Could you check a few things on this model? Use its own coordinates, in mm. Face numbers are marked on the shaded views. A direction names the side the tool comes from. Give positions to 0.01 mm unless a question says otherwise; leave off trailing zeros. Write each loop counter-clockwise with the first axis right and the second up, starting at its lowest first coordinate (ties: lowest second). Pieces come first, ordered by that corner, then holes. Notation, with made-up numbers: (-4, 16.5) - (32, 16.5) arc R10 ccw to (32, 24.5) - close; hole circle Ø2 at (2.25, -33). An arc over 180 degrees is marked (long way). Answer in a Markdown table with one row per item.
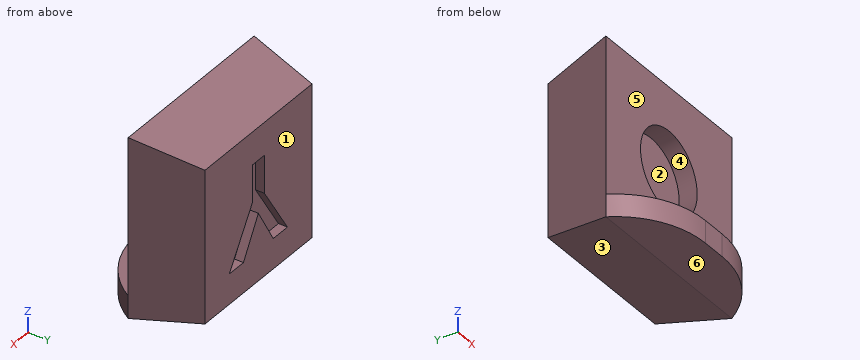
from build123d import *

# Parameters (mm, degrees)
SKETCH1_W               = 8
SKETCH1_H               = 8
BOSS_EXTRUDE1_DEPTH     = 3
CUT_EXTRUDE1_DEPTH      = 12.704699911
CUT_EXTRUDE1_DEPTH_BACK = 12.704699911
CUT_EXTRUDE2_DEPTH      = 11
SKETCH4_R               = 1.8
CUT_EXTRUDE3_DEPTH      = 0.8
SKETCH5_W               = 8
SKETCH5_H               = 1
BOSS_EXTRUDE2_DEPTH     = 2
FILLET1_R               = 4
CUT_EXTRUDE4_DEPTH      = 0.4


with BuildPart() as part:
    # Sketch1 → Boss-Extrude1 (new body)
    with BuildSketch(Plane(origin=(0, 0, 0), x_dir=(1, 0, 0), z_dir=(0, 1, 0))):
        with Locations((4, 4)):
            Rectangle(SKETCH1_W, SKETCH1_H)
    extrude(amount=BOSS_EXTRUDE1_DEPTH)

    # Sketch2 → Cut-Extrude1 (cut, two sides: drawn at the far end of the back side and taken through both)
    with BuildSketch(Plane.XY.offset(-CUT_EXTRUDE1_DEPTH_BACK)):
        Polygon((0, 0), (0.6, 3), (0, 3), align=None)
        Polygon((8, 0), (7.4, 3), (8, 3), align=None)
    extrude(amount=CUT_EXTRUDE1_DEPTH + CUT_EXTRUDE1_DEPTH_BACK, mode=Mode.SUBTRACT)

    # Sketch3 → Cut-Extrude2 (cut)
    with BuildSketch(Plane(origin=(0, 0, 0), x_dir=(0, 0, -1), z_dir=(1, 0, 0))):
        Polygon((0, 0), (0.6, 3), (0, 3), align=None)
        Polygon((8, 3), (7.4, 3), (8, 0), align=None)
    extrude(amount=CUT_EXTRUDE2_DEPTH, mode=Mode.SUBTRACT)

    # Sketch4 → Cut-Extrude3 (cut)
    with BuildSketch(Plane.XZ):
        with Locations(Location((4, -3.75, 0), (0, 0, 270))):
            Circle(SKETCH4_R)
    extrude(amount=-CUT_EXTRUDE3_DEPTH, mode=Mode.SUBTRACT)

    # Sketch5 → Boss-Extrude2 (add)
    with BuildSketch(Plane.XZ):
        with Locations((4, -7.5)):
            Rectangle(SKETCH5_W, SKETCH5_H)
    extrude(amount=BOSS_EXTRUDE2_DEPTH)

    # Fillet1
    # the kernel refuses this fillet: 4 mm, written as the material it takes off along each edge
    with BuildSketch(Plane(origin=(8, -2, -16.660254038), x_dir=(0, 1, 0), z_dir=(0, 0, 1)), Plane(origin=(0, -2, 1.660254038), x_dir=(0, 1, 0), z_dir=(0, 0, -1))) as fillet1_piece_1:
        with BuildLine():
            CenterArc((4, 3.464101615), FILLET1_R, 180, 60)
            Line((0, 3.464101615), (-0.08, 3.464101615))
            Line((-0.08, 3.464101615), (-0.08, 0))
            Line((-0.08, 0), (0, -0.08))
            ThreePointArc((0, -0.08), (1, -0.08), (1.96, -0.069282032))
            Line((1.96, -0.069282032), (2, 0))
        make_face()
    extrude(amount=18.320508076, mode=Mode.SUBTRACT)

    # Sketch6 → Cut-Extrude4 (cut)
    with BuildSketch(Plane(origin=(0, 3, 0), x_dir=(1, 0, 0), z_dir=(0, 1, 0))):
        Polygon((3.623842243, 2.056832464), (3.623842243, 3.740326053), (2.162303782, 6.056832464), (3.062143525, 6.056832464), (4.007656346, 4.408595284), (4.95477173, 6.056832464), (5.854611474, 6.056832464), (4.393073013, 3.734717079), (4.393073013, 2.056832464), align=None)
    extrude(amount=-CUT_EXTRUDE4_DEPTH, mode=Mode.SUBTRACT)


solid = part.part
1) Will these pins go through, and if not, where does the flat tip stop? P1, Ø1, axis at x = 5.5, y = -1.5, coming from the +Z side; P2, Ø3, axis at x = 4.5, z = -4.5, coming from the -Y side.
Check values:
| item | result |
|---|---|
| P1 | stops at z = -7 |
| P2 | stops at y = 0 |
2) On a 3-axis mill with a long thin cutter (end or side, diameter ignored), from which of +Z, -Z, +X, -X, +Y, -Y can I reach the whole of each face in a straight line? I mean the marked faces 5 and 6. Say none if no direction works.
Check values:
| item | result |
|---|---|
| face 5 | +Z, +X, -X, -Y |
| face 6 | -Z, +X, -X, +Y, -Y |
3) Imagine slicing it at A-A (y = 2.7). List the corners of the cut face in (x, z) for me, then the cut area to 3 significant figures.
Check values:
| item | result |
|---|---|
| outline | (0.54, -7.46) - (7.46, -7.46) - (7.46, -0.54) - (0.54, -0.54) - close; hole (2.16, -6.06) - (3.06, -6.06) - (4.01, -4.41) - (4.95, -6.06) - (5.85, -6.06) - (4.39, -3.73) - (4.39, -2.06) - (3.62, -2.06) - (3.62, -3.74) - close |
| area | 43.0 mm2 |
4) Imagine slicing it at B-B (z = -7.25). List the corners of the cut face in (x, y) for me.
Check values:
| item | result |
|---|---|
| outline | (0, 0) arc R4 ccw to (3.46, -2) - (4.54, -2) arc R4 ccw to (8, 0) - (7.4, 3) - (0.6, 3) - close |
5) Imagine slicing it at C-C (x = 6.5). List the corners of the cut face in (y, z) for me, then the cut area to 3 significant figures.
Check values:
| item | result |
|---|---|
| outline | (-1.48, -8) - (0, -8) - (3, -7.4) - (3, -0.6) - (0, 0) - (0, -7) - (-1.48, -7) - close |
| area | 23.7 mm2 |
6) If I drill on line 1 (X direction, y = 2.65, z = -4.75); line 2 (Z direction, x = 4.5, y = -1.05); line 3 (Y direction, x = 7, z = -2.5), over which ranges is the centre line in solid material (lowest first)?
Check values:
| item | result |
|---|---|
| line 1 | x = 0.53 to 2.99, 3.81 to 4.2, 5.03 to 7.47 |
| line 2 | z = -8 to -7 |
| line 3 | y = 0 to 3 |
7) We'd pull the mould along Z, two halves only. Please class the marked faces 1, 2, 3 and 4: +Z half, -Z half, draft (parallel to the pull), parting line (faces both ways), or undercut.
Check values:
| item | result |
|---|---|
| face 1 | draft |
| face 2 | undercut |
| face 3 | -Z half |
| face 4 | undercut |
8) Imagine slicing it at D-D (y = 1.1). List the corners of the cut face in (x, z) for me.
Check values:
| item | result |
|---|---|
| outline | (0.22, -7.78) - (7.78, -7.78) - (7.78, -0.22) - (0.22, -0.22) - close |
